Autodesk Inventor part; units mm, degrees
ref_plane "YZ Plane" through (0, 0, 0) normal (1, 0, 0) x (0, 1, 0)
ref_plane "XZ Plane" through (0, 0, 0) normal (0, 1, 0) x (-1, 0, 0)
ref_plane "XY Plane" through (0, 0, 0) normal (0, 0, 1) x (1, 0, 0)
sketch "Sketch1" plane through (0, 0, 0) normal (0, 1, 0) x (-1, 0, 0)
  line L0 (0, 0) -> (-76.2, 0)
  line L1 (-76.2, 0) -> (-76.2, -76.2)
  line L2 (-76.2, -76.2) -> (0, -76.2)
  line L3 (0, -76.2) -> (0, 0)
  line L4 (-12.7, -2.54) -> (-25.4, -2.54)
  line L5 (-25.4, -2.54) -> (-25.4, -7.366)
  line L6 (-25.4, -7.366) -> (-12.7, -7.366)
  line L7 (-12.7, -7.366) -> (-12.7, -2.54)
  line L8 (-38.1, 0) -> (-38.1, -76.2)
  line L9 (0, -38.1) -> (-76.2, -38.1)
  line L10 (-12.7, -73.66) -> (-25.4, -73.66)
  line L11 (-25.4, -73.66) -> (-25.4, -68.834)
  line L12 (-25.4, -68.834) -> (-12.7, -68.834)
  line L13 (-12.7, -68.834) -> (-12.7, -73.66)
  line L14 (-63.5, -2.54) -> (-50.8, -2.54)
  line L15 (-50.8, -2.54) -> (-50.8, -7.366)
  line L16 (-50.8, -7.366) -> (-63.5, -7.366)
  line L17 (-63.5, -7.366) -> (-63.5, -2.54)
  line L18 (-63.5, -73.66) -> (-50.8, -73.66)
  line L19 (-50.8, -73.66) -> (-50.8, -68.834)
  line L20 (-50.8, -68.834) -> (-63.5, -68.834)
  line L21 (-63.5, -68.834) -> (-63.5, -73.66)
  line L22 (-68.834, -31.75) -> (-68.834, -44.45)
  line L23 (-68.834, -44.45) -> (-73.66, -44.45)
  line L24 (-73.66, -31.75) -> (-68.834, -31.75)
  line L25 (-73.66, -44.45) -> (-73.66, -31.75)
  line L26 (-7.366, -44.45) -> (-2.54, -44.45)
  line L27 (-7.366, -31.75) -> (-7.366, -44.45)
  line L28 (-2.54, -44.45) -> (-2.54, -31.75)
  line L29 (-2.54, -31.75) -> (-7.366, -31.75)
  dimension "d0" = 76.2
  dimension "d1" = 76.2
  dimension "d2" = 12.7
  dimension "d3" = 4.826
  dimension "d4" = 2.54
  dimension "d5" = 12.7
  dimension "d6" = 31.75
  dimension "d7" = 2.54
  dimension "d8" = 4.826
  dimension "d9" = 12.7
extrude "Extrusion1" add sketch "Sketch1" along normal blind 4.826 contours L3 L9 L28 L29 L27 L8 L0 | L8 L9 L22 L24 L25 L1 L0 | L3 L2 L8 L9 L27 L26 L28 | L8 L2 L1 L9 L25 L23 L22
sketch "Sketch3" plane through (0, 4.826, 0) normal (0, 1, 0) x (1, 0, 0)
  arc A0 (62.2366, 56.9773) -> (62.2366, 60.1523) centre (62.2366, 58.5648) ccw
  arc A1 (52.1392, 60.1523) -> (52.1392, 56.9773) centre (52.1392, 58.5648) ccw
  line L0 (62.2366, 60.1523) -> (52.1392, 60.1523)
  line L1 (62.2366, 56.9773) -> (52.1392, 56.9773)
  line L2 (76.2, 0) -> (76.2, 76.2)
  line L3 (76.2, 38.1) -> (0, 38.1)
  line L4 (0, 76.2) -> (0, 0)
  line L5 (76.2, 76.2) -> (0, 76.2)
  line L6 (38.1, 76.2) -> (38.1, 0)
  arc A2 (62.2366, 16.0477) -> (62.2366, 19.2227) centre (62.2366, 17.6352) ccw
  arc A3 (52.1392, 19.2227) -> (52.1392, 16.0477) centre (52.1392, 17.6352) ccw
  line L7 (62.2366, 16.0477) -> (52.1392, 16.0477)
  line L8 (62.2366, 19.2227) -> (52.1392, 19.2227)
  arc A4 (13.9634, 60.1523) -> (13.9634, 56.9773) centre (13.9634, 58.5648) ccw
  arc A5 (24.0608, 56.9773) -> (24.0608, 60.1523) centre (24.0608, 58.5648) ccw
  line L9 (13.9634, 60.1523) -> (24.0608, 60.1523)
  line L10 (13.9634, 56.9773) -> (24.0608, 56.9773)
  arc A6 (13.9634, 19.2227) -> (13.9634, 16.0477) centre (13.9634, 17.6352) ccw
  arc A7 (24.0608, 16.0477) -> (24.0608, 19.2227) centre (24.0608, 17.6352) ccw
  line L11 (13.9634, 16.0477) -> (24.0608, 16.0477)
  line L12 (13.9634, 19.2227) -> (24.0608, 19.2227)
  arc A8 (25.9659, 32.7729) -> (30.7284, 32.7729) centre (28.3471, 32.7729) ccw
  arc A9 (30.7284, 42.5632) -> (25.9659, 42.5632) centre (28.3471, 42.5632) ccw
  line L13 (25.9659, 32.7729) -> (25.9659, 42.5632)
  line L14 (30.7284, 42.5632) -> (30.7284, 32.7729)
  arc A10 (45.4716, 32.7729) -> (50.2341, 32.7729) centre (47.8529, 32.7729) ccw
  arc A11 (50.2341, 42.5632) -> (45.4716, 42.5632) centre (47.8529, 42.5632) ccw
  line L15 (50.2341, 32.7729) -> (50.2341, 42.5632)
  line L16 (45.4716, 42.5632) -> (45.4716, 32.7729)
  dimension "d12" = 3.175
  dimension "d13" = 3.175
  dimension "d16" = 4.7625
  dimension "d17" = 4.7625
extrude "Extrusion3" cut sketch "Sketch3" against normal blind 4.826 contours L1 A1 L0 A0 | L15 A10 L16 L3 | L3 L16 A11 L15 | L14 A8 L13 L3 | L3 L13 A9 L14 | L7 A3 L8 A2 | L9 A5 L10 A4 | L12 A7 L11 A6
fillet "Fillet1" radius 3.175 4 edges at (76.2, 2.413, 0) (76.2, 2.413, -76.2) (0, 2.413, 0) (0, 2.413, -76.2)
properties part number "bottom"
The listing builds one solid part. Answer for the finished solid, in the listing's coordinates (mm). A direction names the side the tool comes from. Coordinates: 2 decimals unless noted, no trailing zeros. Order: outer loops, then holes, each group sorted by start corner. A loop starts at its lowest first (then second) coordinate and runs counter-clockwise, first axis right, second up.
Q1. A cutting plane is placed at B-B, the plane x = 54.5. Write down the section's boundary in (y, z), and give its area (3 significant figures).
Q2. Which of the six approach directions +Z, -Z, +X, -X, +Y, -Y give full straight-line access (tool end or side, diameter ignored) to faces 1 (the face through (30.728, 2, -38)), 2 (the face through (39, 4.826, -38))?
Q3. For a pull along X with two mould halves and no side action, classify faces 3 (the face through (19, 2, -60.152)), 4 (the face through (38, 2, 0)), 5 (the face through (75.25, 2.45, -0.91)) as pulls with the +X half, pulls with the -X half, needs draft (parallel to the pull), parting line crosses it, or undercut.
Q4. A cutting plane is placed at C-C, the plane y = 1.15. State how many separate pieces and enclosed holes the cut face has, and give its area (3 significant figures).
Q5. Consider line 1 (Z direction, x = 62.5, y = 3.3); line 2 (Z direction, x = 55, y = 0.65); line 3 (X direction, y = 0.5, z = -38). Determine where each line is inside the solid, lowest interval first.
Q6. A cutting plane is placed at A-A, the plane z = -38. Write down the section's boundary in (x, y), and give its area (3 significant figures).
Answers follow:
1. outline: (0, -76.2) - (4.83, -76.2) - (4.83, -73.66) - (0, -73.66) - close; (0, -68.83) - (4.83, -68.83) - (4.83, -60.15) - (0, -60.15) - close; (0, -56.98) - (4.83, -56.98) - (4.83, -19.22) - (0, -19.22) - close; (0, -16.05) - (4.83, -16.05) - (4.83, -7.37) - (0, -7.37) - close; (0, -2.54) - (4.83, -2.54) - (4.83, 0) - (0, 0) - close
1. area: 291 mm2
2. face 1: +Y, -Y
2. face 2: +Z, -Z, +X, -X, +Y
3. face 3: undercut
3. face 4: needs draft
3. face 5: pulls with the +X half
4. separate pieces: 1
4. enclosed holes: 12
4. area: 5,140 mm2
5. line 1: z = -76.2 to -73.66, -68.83 to -60.13, -57 to -19.2, -16.07 to -7.37, -2.54 to 0
5. line 2: z = -76.2 to -73.66, -68.83 to -60.15, -56.98 to -19.22, -16.05 to -7.37, -2.54 to 0
5. line 3: x = 0 to 2.54, 7.37 to 25.97, 30.73 to 45.47, 50.23 to 68.83, 73.66 to 76.2
6. outline: (0, 0) - (2.54, 0) - (2.54, 4.83) - (0, 4.83) - close; (7.37, 0) - (25.97, 0) - (25.97, 4.83) - (7.37, 4.83) - close; (30.73, 0) - (45.47, 0) - (45.47, 4.83) - (30.73, 4.83) - close; (50.23, 0) - (68.83, 0) - (68.83, 4.83) - (50.23, 4.83) - close; (73.66, 0) - (76.2, 0) - (76.2, 4.83) - (73.66, 4.83) - close
6. area: 275 mm2
